Check sheet for the drawn part. Datum: minimum x, y, z corner. Units: mm. Give positions to 0.01 mm unless a question says otherwise; leave off trailing zeros. Loops run counter-clockwise (first coordinate to the right, second up) from the corner with the lowest first, then second, coordinate; pieces in that order, holes last. Notation, with made-up numbers: M 8,-2 L 53,-2 A35 ccw 53,32 Z; hole C -8,62.5 d2. An arc over 180 degrees is marked long. Write each question's results on one line, items separated by ' | '. Start each with the question number.
1. Material ranges on line 1 along X through (y, z) = (1.9, 15.5); line 2 along Z through (x, y) = (71.05, 1.2); line 3 along X through (y, z) = (9.5, 25.5), recorded low to high.
2. Go/stop test with flat-tipped pins: pin 1 (6.5 mm diameter, centred on y = 10.5, z = 20, fed in from +X); pin 2 (1 mm diameter, centred on y = 18, z = 23.5, fed in from -X); pin 3 (1.4 mm diameter, centred on x = 3.5, y = 2, fed in from -Z); pin 4 (3.5 mm diameter, centred on x = 4.55, z = 15.5, fed in from +Y). Record where each tip stops, or that it passes through.
3. Sectioned sample at A-A on z = 15.5. Record the cut outline in (x, y), and give its area (3 significant figures).
4. Sectioned sample at D-D on z = 6. Record the cut outline in (x, y).
5. Sectioned sample at C-C on y = 16.5. Record the cut outline in (x, z), and give its area (3 significant figures).
6. Sectioned sample at B-B on x = 4.55. Record the cut outline in (y, z), and give its area (3 significant figures).
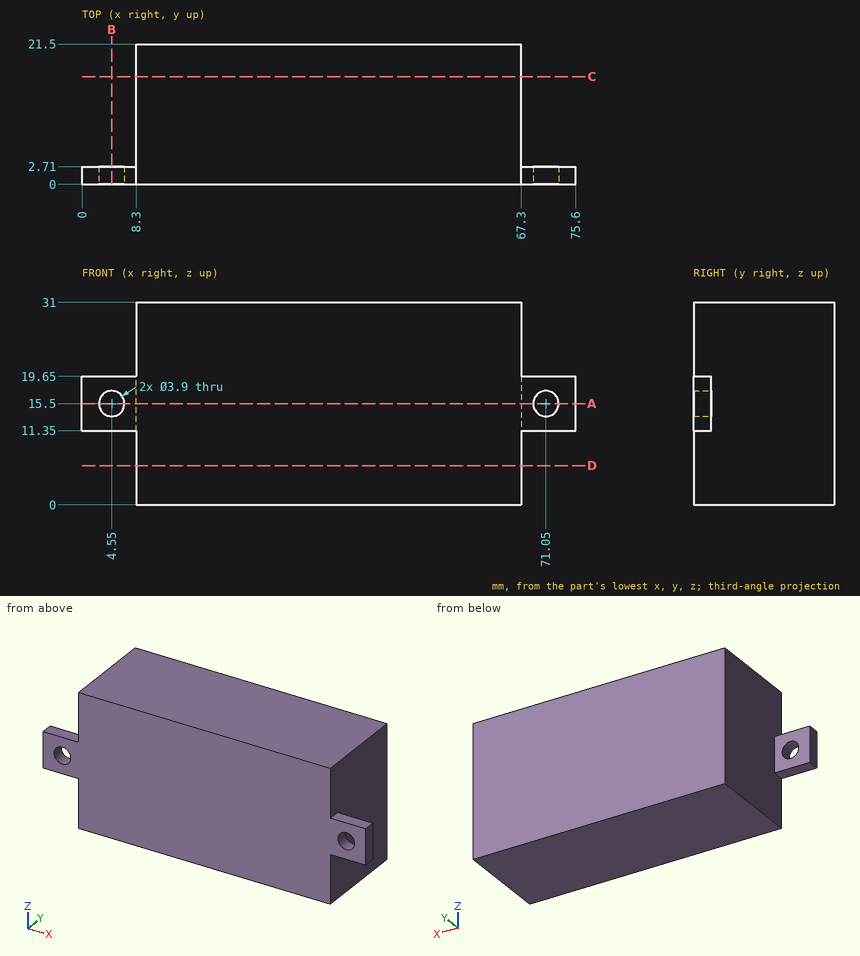
Output values:
1) line 1: 0 to 2.6, 6.5 to 69.1, 73 to 75.6 | line 2: 11.35 to 13.55, 17.45 to 19.65 | line 3: 8.3 to 67.3
2) pin 1: x = 67.3 | pin 2: x = 8.3 | pin 3: z = 11.35 | pin 4: through
3) outline: M 0,0 L 2.6,0 L 2.6,2.71 L 0,2.71 Z; M 6.5,0 L 69.1,0 L 69.1,2.71 L 67.3,2.71 L 67.3,21.5 L 8.3,21.5 L 8.3,2.71 L 6.5,2.71 Z; M 73,0 L 75.6,0 L 75.6,2.71 L 73,2.71 Z | area: 1,290 mm2
4) outline: M 8.3,0 L 67.3,0 L 67.3,21.5 L 8.3,21.5 Z
5) outline: M 8.3,0 L 67.3,0 L 67.3,31 L 8.3,31 Z | area: 1,830 mm2
6) outline: M 0,11.35 L 2.71,11.35 L 2.71,13.55 L 0,13.55 Z; M 0,17.45 L 2.71,17.45 L 2.71,19.65 L 0,19.65 Z | area: 11.9 mm2
